Check sheet for the modelled part. Datum: model origin and axes. Units: mm. A direction names the side the tool comes from. Coordinates: 2 decimals unless noted, no trailing zeros. Loops run counter-clockwise (first coordinate to the right, second up) from the corner with the lowest first, then second, coordinate; pieces in that order, holes last.
```python
from build123d import *

# Parameters (mm, degrees)
F0_W     = 64.7562947124
F0_H     = 50.6538115442
F1_DEPTH = 25.4
F2_R     = 11.1559539437
F3_DEPTH = 50.292
F4_R     = 18.0527377002
F4_R_2   = 11.1559539437
F5_DEPTH = 13.97


with BuildPart() as f1:
    # F0 (on Front) → F1 (new body)
    with BuildSketch(Plane.XZ):
        with Locations((3.1658643857, 2.158543095)):
            Rectangle(F0_W, F0_H)
    extrude(amount=F1_DEPTH)

    # F2 (on face) → F3 (cut)
    with BuildSketch(Plane.XZ.offset(25.4)):
        Circle(F2_R)
    extrude(amount=-F3_DEPTH, mode=Mode.SUBTRACT)

    # F4 (on face) → F5 (join)
    with BuildSketch(Plane.XZ.offset(25.4)):
        Circle(F4_R)
        Circle(F4_R_2, mode=Mode.SUBTRACT)
    extrude(amount=F5_DEPTH)


solid = f1.part
```
1) Section check B-B on x = 0. Enter the section's corners in (y, z), plus the area to 3 significant figures.
Answer sheet:
outline: (-39.37, -18.05) - (-25.4, -18.05) - (-25.4, -23.17) - (0, -23.17) - (0, -11.16) - (-39.37, -11.16) - close; (-39.37, 11.16) - (0, 11.16) - (0, 27.49) - (-25.4, 27.49) - (-25.4, 18.05) - (-39.37, 18.05) - close
area: 913 mm2
2) Scan lines: line 1 (Z direction, x = 0, y = -34.5); line 2 (Z direction, x = 0, y = -13); line 3 (Y direction, x = -13.5, z = 13.5). Record each from-to range of solid material in increasing order.
Answer sheet:
line 1: z = -18.05 to -11.16, 11.16 to 18.05
line 2: z = -23.17 to -11.16, 11.16 to 27.49
line 3: y = -25.4 to 0
3) Set-up check for faces 1 (the flat face through (-29.212, -13, 2)), 2 (the flat face through (17, -25.4, 8)): record each of +Z, -Z, +X, -X, +Y, -Y from which the full face is reachable in a straight line by a thin tool's end or side.
Answer sheet:
face 1: +Z, -Z, -X, +Y, -Y
face 2: -Y
4) Section check D-D on x = 13.5. Enter the section's corners in (y, z).
Answer sheet:
outline: (-39.37, -11.99) - (-25.4, -11.99) - (-25.4, -23.17) - (0, -23.17) - (0, 27.49) - (-25.4, 27.49) - (-25.4, 11.99) - (-39.37, 11.99) - close
5) Section check A-A on z = 0. Enter the section's corners in (x, y), plus the area to 3 significant figures.
Answer sheet:
outline: (-29.21, -25.4) - (-18.05, -25.4) - (-18.05, -39.37) - (-11.16, -39.37) - (-11.16, 0) - (-29.21, 0) - close; (11.16, -39.37) - (18.05, -39.37) - (18.05, -25.4) - (35.54, -25.4) - (35.54, 0) - (11.16, 0) - close
area: 1,270 mm2
6) Depth check by flat-ended pin: pin 1 (2 mm diameter, centred on y = -26.5, z = 13, fed in from +X); pin 2 (20 mm diameter, centred on x = 0, z = 0, fed in from +Y). Enter the tip coordinate at first touch or a pass-through.
Answer sheet:
pin 1: stops at x = 13.49
pin 2: passes through
7) Section check C-C on y = -19.5. Enter the section's corners in (x, z), plus the area to 3 significant figures.
Answer sheet:
outline: (-29.21, -23.17) - (35.54, -23.17) - (35.54, 27.49) - (-29.21, 27.49) - close; hole circle Ø22.31 at (0, 0)
area: 2,890 mm2
